from build123d import *

# Parameters (mm, degrees)
SKETCH1_R           = 1.5
SKETCH1_W           = 22.5
SKETCH1_H           = 12.2
BOSS_EXTRUDE1_DEPTH = 5
SKETCH2_R           = 15
BOSS_EXTRUDE2_DEPTH = 5


with BuildPart() as part:
    # Sketch1 → Boss-Extrude1 (new body)
    with BuildSketch(Plane.XY):
        Polygon((0, 0), (-55, 0), (-55, 39.4), (0, 39.4), (0, 15), (20, 15), (20, 0), align=None)
        with Locations((12.5, 7.5)):
            Circle(SKETCH1_R, mode=Mode.SUBTRACT)
        with Locations((-38.75, 11.1)):
            Rectangle(SKETCH1_W, SKETCH1_H, mode=Mode.SUBTRACT)
        with Locations((-16.25, 28.3)):
            Rectangle(SKETCH1_W, SKETCH1_H, mode=Mode.SUBTRACT)
    extrude(amount=BOSS_EXTRUDE1_DEPTH)

    # Sketch2 → Boss-Extrude2 (add)
    with BuildSketch(Plane.XZ):
        with Locations((-35, 1.929670276)):
            Circle(SKETCH2_R)
    extrude(amount=BOSS_EXTRUDE2_DEPTH)


solid = part.part
Model file for the job. Use its own axes, mm. A direction names the side the tool comes from. Round coordinates to 2 decimals unless told otherwise and drop trailing zeros. Loops run counter-clockwise (first coordinate to the right, second up) from the corner with the lowest first, then second, coordinate; pieces in that order, holes last. Notation, with made-up numbers: M -9.75,26 L 18.25,26 A14 cw 18.25,52 Z; hole C 1.25,61.25 d11. An arc over 180 degrees is marked long. One line per question, with ' | ' between items.
1) Mould opens along X. For faces 5 (the flat face through (-27.5, 11, 2)), 6 (the cylindrical face through (-49.985, -2.465, 2.589)), 7 (the flat face through (-52, 0, 2)) say: +X half, -X half, draft (parallel to the pull), parting line (faces both ways), or undercut.
Solved:
face 5: undercut | face 6: parting line | face 7: draft
2) Band-saw the part on A-A (y = 7.5). Give the cut face in (x, z).
Solved:
outline: M -55,0 L -50,0 L -50,5 L -55,5 Z; M -27.5,0 L 11,0 L 11,5 L -27.5,5 Z; M 14,0 L 20,0 L 20,5 L 14,5 Z
3) Band-saw the part on C-C (x = 12.5). Give the cut face in (y, z).
Solved:
outline: M 0,0 L 6,0 L 6,5 L 0,5 Z; M 9,0 L 15,0 L 15,5 L 9,5 Z
4) Band-saw the part on B-B (x = -10). Give the cut face in (y, z).
Solved:
outline: M 0,0 L 22.2,0 L 22.2,5 L 0,5 Z; M 34.4,0 L 39.4,0 L 39.4,5 L 34.4,5 Z
5) Drill centre lines: line 1 along Y through (x, z) = (12.5, 2.5); line 2 along Z through (x, y) = (-24, 5); line 3 along Y through (x, z) = (-43, 11.5). Where is each one in solid material? Low to high.
Solved:
line 1: y = 0 to 6, 9 to 15 | line 2: z = 0 to 5 | line 3: y = -5 to 0
6) Flat gauge pins, fed straight in: pin 1 (10 mm diameter, centred on x = 1.5, y = 16, fed in from -Z); pin 2 (2.5 mm diameter, centred on y = 25, z = 3, fed in from +X); pin 3 (5 mm diameter, centred on y = 1.5, z = 9.5, fed in from -X); pin 4 (6 mm diameter, centred on x = 5.5, z = -3.5, fed in from -Y). Where does each tip first touch, or does it go through?
Solved:
pin 1: stops at z = 0 | pin 2: stops at x = 0 | pin 3: stops at x = -48.93 | pin 4: passes through
7) Band-saw the part on D-D (y = 37). Give the cut face in (x, z), then the cut area to 3 significant figures.
Solved:
outline: M -55,0 L 0,0 L 0,5 L -55,5 Z | area: 275 mm²
8) 3-axis set-ups, long thin cutter, end or side, ignore diameter. For faces 1 (the flat face through (-35, 0, 10)), 2 (the flat face through (10, 15, 2)), 3 (the flat face through (-25, 20, 0)), 4 (the flat face through (-50, 11, 2)): which of +Z, -Z, +X, -X, +Y, -Y reach the whole face in a straight line?
Solved:
face 1: +Z, +X, -X, +Y | face 2: +Z, -Z, +X, +Y | face 3: -Z, +X, -X, +Y | face 4: +Z, -Z
